```python
from build123d import *

# Parameters (mm, degrees)
SKETCH2_W           = 37
SKETCH2_H           = 50
SKETCH2_W_2         = 32
SKETCH2_H_2         = 43.243243244
BOSS_EXTRUDE1_DEPTH = 25
SKETCH4_W           = 37
SKETCH4_H           = 50
BOSS_EXTRUDE2_DEPTH = 5
SKETCH5_R           = 4.7
CUT_EXTRUDE1_DEPTH  = 65
SKETCH6_R           = 1.15
BOSS_EXTRUDE3_DEPTH = 4
SKETCH7_R           = 1.7
BOSS_EXTRUDE4_DEPTH = 3


with BuildPart() as part:
    # Sketch2 → Boss-Extrude1 (new body)
    with BuildSketch(Plane(origin=(0, 0, 0), x_dir=(1, 0, 0), z_dir=(0, 1, 0))):
        Rectangle(SKETCH2_W, SKETCH2_H)
        Rectangle(SKETCH2_W_2, SKETCH2_H_2, mode=Mode.SUBTRACT)
    extrude(amount=BOSS_EXTRUDE1_DEPTH)

    # Sketch4 → Boss-Extrude2 (add)
    with BuildSketch(Plane.XZ):
        Rectangle(SKETCH4_W, SKETCH4_H)
    extrude(amount=BOSS_EXTRUDE2_DEPTH)

    # Sketch5 → Cut-Extrude1 (cut)
    with BuildSketch(Plane(origin=(0, 0, -25), x_dir=(-1, 0, 0), z_dir=(0, 0, -1))):
        with Locations((0, 10)):
            Circle(SKETCH5_R)
    extrude(amount=-CUT_EXTRUDE1_DEPTH, mode=Mode.SUBTRACT)

    # Sketch6 → Boss-Extrude3 (add)
    with BuildSketch(Plane(origin=(0, 25, 0), x_dir=(1, 0, 0), z_dir=(0, 1, 0))):
        with Locations(Location((-16.7, 23.25, 0), (0, 0, 270))):
            Circle(SKETCH6_R)
        with Locations(Location((16.7, 23.25, 0), (0, 0, 90))):
            Circle(SKETCH6_R)
        with Locations(Location((16.7, -23.25, 0), (0, 0, 270))):
            Circle(SKETCH6_R)
        with Locations(Location((-16.7, -23.25, 0), (0, 0, 90))):
            Circle(SKETCH6_R)
    extrude(amount=BOSS_EXTRUDE3_DEPTH)

    # Sketch7 → Boss-Extrude4 (add)
    with BuildSketch(Plane.XZ.offset(5)):
        Polygon((-18.5, 0), (-18.5, 3), (-24.5, 3), (-24.5, -3), (-18.5, -3), align=None)
        with Locations(Location((-21.5, 0, 0), (0, 0, 270))):
            Circle(SKETCH7_R, mode=Mode.SUBTRACT)
    boss_extrude4 = extrude(amount=-BOSS_EXTRUDE4_DEPTH)

    # Mirror1: Boss-Extrude4 across plane
    add(boss_extrude4.mirror(Plane(origin=(0, 0, 0), x_dir=(0, 0, 1), z_dir=(1, 0, 0))))


solid = part.part
```
CAD build for the part. Positions are in the model's coordinates, mm. A direction names the side the tool comes from. Round coordinates to 2 decimals unless told otherwise and drop trailing zeros. Order: outer loops, then holes, each group sorted by start corner. A loop starts at its lowest first (then second) coordinate and runs counter-clockwise, first axis right, second up.
Item 1: Pin check, flat tips, straight feed: pin 1 (9 mm diameter, centred on y = 3.5, z = 4, fed in from +X); pin 2 (3.5 mm diameter, centred on x = -21, y = -3.5, fed in from +Z); pin 3 (1.5 mm diameter, centred on y = 0, z = -7, fed in from -X). Stop position of each tip, or through.
Item 2: Saw through at A-A on x = -21.5. Write the cut outline in (y, z), then the cut area to 3 significant figures.
Item 3: Probe line 1 along X through (y, z) = (-3.5, 0); line 2 along Z through (x, y) = (-13.5, 20); line 3 along Y through (x, z) = (0, 22). List the from-to ranges inside material, lowest first.
Item 4: Mould opens along X. For faces 1 (the face through (-4, 7, -25)), 2 (the face through (16, 12, 0)) say: pulls with the +X half, pulls with the -X half, needs draft (parallel to the pull), parting line crosses it, or undercut.
Item 5: Saw through at B-B on z = -23.25. Write the cut outline in (x, y).
Item 6: Saw through at C-C on x = 0. Write the cut outline in (y, z), then the cut area to 3 significant figures.
Item 7: Saw through at D-D on z = 0. Write the cut outline in (x, y).
Item 8: Tool access for faces 3 (the face through (-21, -4, 3)), 4 (the face through (16.2, 25, -0.4)), 5 (the face through (22, -4, -3)), 6 (the face through (-22.9, -2, -1.3)): list every direction of +Z, -Z, +X, -X, +Y, -Y with a clear straight run to the whole face (end or side of a thin tool).
Reported:
1. pin 1: stops at x = 18.5
1. pin 2: stops at z = 3
1. pin 3: stops at x = -18.5
2. outline: (-5, -3) - (-2, -3) - (-2, -1.7) - (-5, -1.7) - close; (-5, 1.7) - (-2, 1.7) - (-2, 3) - (-5, 3) - close
2. area: 7.80 mm2
3. line 1: x = -24.5 to -23.2, -19.8 to 19.8, 23.2 to 24.5
3. line 2: z = -25 to -21.62, 21.62 to 25
3. line 3: y = -5 to 5.3, 14.7 to 25
4. face 1: needs draft
4. face 2: undercut
5. outline: (-18.5, -5) - (18.5, -5) - (18.5, 25) - (17.85, 25) - (17.85, 29) - (15.55, 29) - (15.55, 25) - (-15.55, 25) - (-15.55, 29) - (-17.85, 29) - (-17.85, 25) - (-18.5, 25) - close; hole circle Ø9.4 at (0, 10)
6. outline: (-5, -25) - (5.3, -25) - (5.3, -21.62) - (0, -21.62) - (0, 21.62) - (5.3, 21.62) - (5.3, 25) - (-5, 25) - close; (14.7, -25) - (25, -25) - (25, -21.62) - (14.7, -21.62) - close; (14.7, 21.62) - (25, 21.62) - (25, 25) - (14.7, 25) - close
6. area: 355 mm2
7. outline: (-24.5, -5) - (-23.2, -5) - (-23.2, -2) - (-24.5, -2) - close; (-19.8, -5) - (19.8, -5) - (19.8, -2) - (18.5, -2) - (18.5, 25) - (16, 25) - (16, 0) - (-16, 0) - (-16, 25) - (-18.5, 25) - (-18.5, -2) - (-19.8, -2) - close; (23.2, -5) - (24.5, -5) - (24.5, -2) - (23.2, -2) - close
8. face 3: +Z, -X, +Y, -Y
8. face 4: +Y
8. face 5: -Z, +X, +Y, -Y
8. face 6: +Z, -Z, -X, +Y
